from build123d import *

# Parameters (mm, degrees)
F0_W        = 25
F0_H        = 40
F1_DEPTH    = 25
F0_R        = 2
F2_DEPTH    = 3
F3_SIZE     = 5
F4_SIZE     = 5
F5_T        = 3
F5_T3_DEPTH = 21
F5_T5_DEPTH = 13.0710678119
F5_T7_DEPTH = 13.0710678119


# Not quite as in the source:
# - a shell that OpenCascade refuses in one call is made with other operations: the cavity is built on its own and cut out


with BuildPart() as f1:
    # F0 (on Top) → F1 (new body)
    with BuildSketch(Plane.XY):
        Rectangle(F0_W, F0_H)
    extrude(amount=F1_DEPTH)

    # F0 (on Top) → F2 (join)
    with BuildSketch(Plane.XY):
        with BuildLine():
            Line((-3.6435657461, 29.4240953044), (-12.5, 20))
            Line((-12.5, 20), (12.5, 20))
            Line((12.5, 20), (3.6435657461, 29.4240953044))
            ThreePointArc((3.6435657461, 29.4240953044), (4.6485389495, 27.8414900583), (5, 26))
            ThreePointArc((5, 26), (-1.8414900583, 21.3514610505), (-3.6435657461, 29.4240953044))
        make_face()
        with BuildLine():
            ThreePointArc((3.6435657461, 29.4240953044), (0, 31), (-3.6435657461, 29.4240953044))
            ThreePointArc((-3.6435657461, 29.4240953044), (-1.8414900583, 21.3514610505), (5, 26))
            ThreePointArc((5, 26), (4.6485389495, 27.8414900583), (3.6435657461, 29.4240953044))
        make_face()
        with Locations((0, 26)):
            Circle(F0_R, mode=Mode.SUBTRACT)
    extrude(amount=F2_DEPTH)

    # F3
    f3_edges = [f1.edges().sort_by_distance(p)[0] for p in [
        (12.5, 0, 25),
        (0, -20, 25),
        (-12.5, 0, 25),
        (0, 20, 25),
    ]]
    chamfer(f3_edges, length=F3_SIZE)

    # F4
    f4_edges = [f1.edges().sort_by_distance(p)[0] for p in [
        (-12.5, -20, 10),
        (12.5, -20, 10),
        (12.5, 20, 11.5),
        (-12.5, 20, 11.5),
    ]]
    chamfer(f4_edges, length=F4_SIZE)

    # F5: shell of thickness 3, made by hand


with BuildPart() as f5_core1:
    # F5_t2: copy of F1
    add(f1.part)

    # the walls: a layer under each face that stays
    f5_faces = [f5_core1.faces().sort_by_distance(p)[0] for p in [
        (0, 20, 11.5),
        (0, 17.5, 22.5),
        (10, 17.5, 12.75),
        (-10, 17.5, 12.75),
        (0, 23, 3),
        (10, 0, 22.5),
        (0, 0, 25),
        (-10, 0, 22.5),
        (12.5, 2.5, 10),
        (-12.5, 2.5, 10),
        (-8.0717828731, 24.7120476522, 1.5),
        (8.0717828731, 24.7120476522, 1.5),
        (0, 31, 1.5),
        (-2, 26, 1.5),
        (0, -17.5, 22.5),
        (10, -17.5, 11.25),
        (-10, -17.5, 11.25),
        (0, -20, 10),
    ]]
    thicken(f5_faces, amount=-F5_T, mode=Mode.SUBTRACT)

    # F5_s4 → F5_t3 (cut)
    with BuildSketch(Plane.YZ.offset(-10.5)):
        Polygon((20.03, 3.03), (17, 3), (17, 0), (20, 0), align=None)
    extrude(amount=F5_T3_DEPTH, mode=Mode.SUBTRACT)

    # F5_s6 → F5_t5 (cut)
    with BuildSketch(Plane(origin=(-8.3713203436, 8.3713203436, 0), x_dir=(0, 0, 1), z_dir=(0.7071067812, -0.7071067812, 0))):
        Polygon((3.03, -19.4754364826), (3, -16.4454364826), (0, -16.4454364826), (0, -19.4454364826), align=None)
    extrude(amount=F5_T5_DEPTH, mode=Mode.SUBTRACT)

    # F5_s8 → F5_t7 (cut)
    with BuildSketch(Plane(origin=(8.3713203436, 8.3713203436, 0), x_dir=(0, 0, 1), z_dir=(-0.7071067812, -0.7071067812, 0))):
        Polygon((3.03, 19.4754364826), (3, 16.4454364826), (0, 16.4454364826), (0, 19.4454364826), align=None)
    extrude(amount=F5_T7_DEPTH, mode=Mode.SUBTRACT)


with BuildPart() as f1_1:
    add(f1.part)

    # what is left inside the walls is the cavity
    f5_cavity = [f5_core1.part.solids().sort_by_distance(p)[0] for p in [
        (0, -5.666667, 0.03),
    ]]
    add(f5_cavity, mode=Mode.SUBTRACT)


solid = f1_1.part
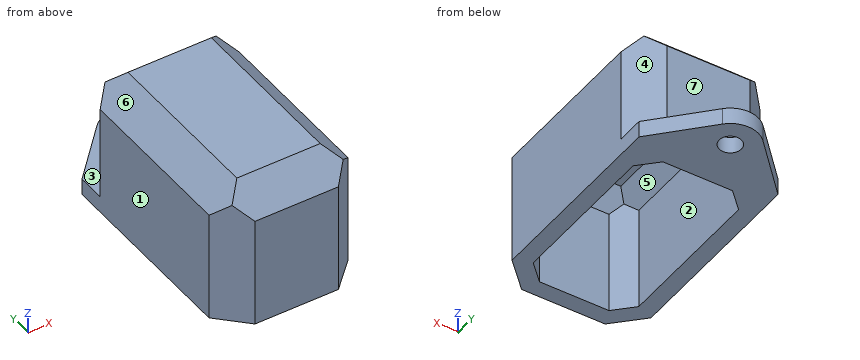
Geometry: final body of the model. Coordinates: model frame, mm. Face numbers are marked on the shaded views. A direction names the side the tool comes from. Round coordinates to 2 decimals unless told otherwise and drop trailing zeros. Write each loop counter-clockwise with the first axis right and the second up, starting at its lowest first coordinate (ties: lowest second). Pieces come first, ordered by that corner, then holes. Notation, with made-up numbers: M 32,-17.5 L 75,-17.5 A34 ccw 75,15.5 Z; hole C 89,11 d9. An arc over 180 degrees is marked long. Write item = value, one per line.
Item 1: Access query for the marked faces 4, 5, 6 and 7. Directions: +Z, -Z, +X, -X, +Y, -Y. A direction counts if a zero-diameter tool reaches every point of the face in a straight line with its end or side. Return the directions, or none.
Findings:
face_4 = +Z, +X, +Y
face_5 = -Z
face_6 = +Z, -X, +Y, -Y
face_7 = +Z, +X, -X, +Y
Item 2: Material intervals for line 1 along Y through (x, z) = (0, 1.5); line 2 along Y through (x, z) = (5.75, 12.5); line 3 along X through (y, z) = (1.5, 1), sorted ascending. Write a range as [from, to].
Findings:
line_1 = [-20, -17], [17, 24], [28, 31]
line_2 = [-20, -17], [17, 20]
line_3 = [-12.5, -9.5], [9.5, 12.5]
Item 3: Section query C-C on y = -1.5. Return loops of the section in (x, z), then the cut area to 3 significant figures.
Findings:
outline = M -12.5,0 L -9.5,0 L -9.5,18.76 L -6.26,22 L 6.26,22 L 9.5,18.76 L 9.5,0 L 12.5,0 L 12.5,20 L 7.5,25 L -7.5,25 L -12.5,20 Z
area = 193 mm^2
Item 4: Section query B-B on x = 0. Return loops of the section in (y, z).
Findings:
outline = M -20,0 L -17,0 L -17,18.76 L -13.76,22 L 13.76,22 L 17,18.76 L 17,0 L 24,0 L 24,3 L 20,3 L 20,20 L 15,25 L -15,25 L -20,20 Z; M 28,0 L 31,0 L 31,3 L 28,3 Z
Item 5: Pin query (flat end, axial travel): P1, Ø10, axis at x = -2.5, y = -0.5, coming from the -Z side; P2, Ø5, axis at x = -5.5, z = 19, coming from the +Y side; P3, Ø4, axis at y = 18, z = 7.5, coming from the +X side; P4, Ø3, axis at x = 0, y = 26, coming from the +Z side. Return the tip coordinate at first contact, or that it passes through.
Findings:
P1 = 20.76
P2 = 20
P3 = 11.5
P4 = through
Item 6: Section query A-A on z = 5.75. Return loops of the section in (x, y), then the cut area to 3 significant figures.
Findings:
outline = M -12.5,-15 L -7.5,-20 L 7.5,-20 L 12.5,-15 L 12.5,15 L 7.5,20 L -7.5,20 L -12.5,15 Z; hole M -9.5,-13.76 L -6.26,-17 L 6.26,-17 L 9.5,-13.76 L 9.5,13.76 L 6.26,17 L -6.26,17 L -9.5,13.76 Z
area = 325 mm^2
Item 7: Pull-direction query (X, two-part tool) for the marked faces 1, 2 and 3; classes: pulls with the +X half, pulls with the -X half, needs draft (parallel to the pull), parting line crosses it, or undercut.
Findings:
face_1 = pulls with the -X half
face_2 = undercut
face_3 = needs draft
Item 8: Section query D-D on y = 27. Return loops of the section in (x, z).
Findings:
outline = M -5.92,0 L -1.73,0 L -1.73,3 L -5.92,3 Z; M 1.73,0 L 5.92,0 L 5.92,3 L 1.73,3 Z
